from build123d import *

# Parameters (mm, degrees)
SKETCH_398_R        = 1.75
EXTRUDE_1_DEPTH     = 4
CHAMFER_1_SIZE      = 1.5
SKETCH_632_W        = 24
SKETCH_632_H        = 16
SKETCH_632_R        = 1.6
CUT_EXTRUDE_1_DEPTH = 3
SKETCH_910_R        = 2.5
SKETCH_910_W        = 7
SKETCH_910_H        = 4
EXTRUDE_2_DEPTH     = 1.2
SKETCH_1130_R       = 1.2
CUT_EXTRUDE_2_DEPTH = 0.7
CHAMFER_2_SIZE      = 1.2
CHAMFER_3_SIZE      = 2


with BuildPart() as part:
    # Sketch 398 → Бобышка-Вытянуть1 (new body)
    with BuildSketch(Plane(origin=(0, 0, 0), x_dir=(1, 0, 0), z_dir=(0, 1, 0))):
        with BuildLine():
            Line((-15, 4), (-13.5, 4))
            Line((-13.5, 4), (-13.5, 9.5))
            Line((-13.5, 9.5), (13.5, 9.5))
            Line((13.5, 9.5), (13.5, 4))
            Line((13.5, 4), (15, 4))
            ThreePointArc((15, 4), (19, 0), (15, -4))
            Line((15, -4), (13.5, -4))
            Line((13.5, -4), (13.5, -9.5))
            Line((13.5, -9.5), (-13.5, -9.5))
            Line((-13.5, -9.5), (-13.5, -4))
            Line((-13.5, -4), (-15, -4))
            ThreePointArc((-15, -4), (-19, 0), (-15, 4))
        make_face()
        with Locations((-15, 0)):
            Circle(SKETCH_398_R, mode=Mode.SUBTRACT)
        with Locations((15, 0)):
            Circle(SKETCH_398_R, mode=Mode.SUBTRACT)
    extrude(amount=EXTRUDE_1_DEPTH)

    # Фаска1
    chamfer_1_edges = [part.edges().sort_by_distance(p)[0] for p in [
        (13.25, 0, 0),
        (-16.75, 0, 0),
    ]]
    chamfer(chamfer_1_edges, length=CHAMFER_1_SIZE)

    # Sketch 632 → Вырез-Вытянуть1 (cut)
    with BuildSketch(Plane(origin=(0, 4, 0), x_dir=(1, 0, 0), z_dir=(0, 1, 0))):
        Rectangle(SKETCH_632_W, SKETCH_632_H)
        with Locations((-2.8, 4.2)):
            Circle(SKETCH_632_R, mode=Mode.SUBTRACT)
        with Locations((-2.8, -4.2)):
            Circle(SKETCH_632_R, mode=Mode.SUBTRACT)
    extrude(amount=-CUT_EXTRUDE_1_DEPTH, mode=Mode.SUBTRACT)

    # Sketch 910 → Бобышка-Вытянуть2 (add)
    with BuildSketch(Plane(origin=(0, 1, 0), x_dir=(1, 0, 0), z_dir=(0, 1, 0))):
        with Locations((-2.8, -4.2)):
            Circle(SKETCH_910_R)
        with Locations((-2.8, 4.2)):
            Circle(SKETCH_910_R)
        with Locations((8.5, -6)):
            Rectangle(SKETCH_910_W, SKETCH_910_H)
        with Locations((8.5, 6)):
            Rectangle(SKETCH_910_W, SKETCH_910_H)
    extrude(amount=EXTRUDE_2_DEPTH)

    # Sketch 1130 → Вырез-Вытянуть2 (cut)
    with BuildSketch(Plane(origin=(0, 1, 0), x_dir=(1, 0, 0), z_dir=(0, 1, 0))):
        with Locations((-8.3, 5.4)):
            Circle(SKETCH_1130_R)
    extrude(amount=-CUT_EXTRUDE_2_DEPTH, mode=Mode.SUBTRACT)

    # Фаска2
    chamfer_2_edges = [part.edges().sort_by_distance(p)[0] for p in [
        (12, 1, 0),
        (-3.5, 1, -8),
        (-12, 1, 0),
        (-3.5, 1, 8),
    ]]
    chamfer(chamfer_2_edges, length=CHAMFER_2_SIZE)

    # Фаска3
    chamfer_3_edges = [part.edges().sort_by_distance(p)[0] for p in [
        (0, 0, -9.5),
        (13.5, 0, -6.75),
        (13.5, 0, 6.75),
        (0, 0, 9.5),
        (-13.5, 0, 6.75),
        (-13.5, 0, -6.75),
    ]]
    chamfer(chamfer_3_edges, length=CHAMFER_3_SIZE)


solid = part.part
Read the model definition and answer for the solid it produces. Units are mm, in the model's axes. A direction names the side the tool comes from. Coordinates: 2 decimals unless noted, no trailing zeros. Order: outer loops, then holes, each group sorted by start corner. A loop starts at its lowest first (then second) coordinate and runs counter-clockwise, first axis right, second up. Notation, with made-up numbers: M 49.5,81.25 L 104.5,81.25 A19 cw 104.5,109.25 Z; hole C -6.75,-35 d7. An arc over 180 degrees is marked long. Put each result on its own line as item: value. Start each with the question number.
Item 1: Section A-A, the plane y = 2.55 is taken. Determine the outline of the cut face in (x, z), plus the area to 3 significant figures.
Item 2: Section D-D, the plane z = 0.5 is taken. Count the separate pieces of the cut face and the enclosed holes in it, plus the area to 3 significant figures.
Item 3: The mould has two halves that part along X. Classify faces 1 (the face through (5, 2, -6)), 2 (the face through (13.5, 3, -7)), 3 (the face through (-12.5, 1, -6.1)): +X half, -X half, draft (parallel to the pull), parting line (faces both ways), or undercut.
Item 4: Consider probe 1 along X at (y, z) = (2.25, 0); probe 2 along X at (y, z) = (2.25, 7); probe 3 along X at (y, z) = (1.55, -0.25). Determine where each line is inside the solid, lowest interval first. Write a range as [from, to].
Item 5: Section B-B, the plane x = -8.3 is taken. Determine the outline of the cut face in (y, z), plus the area to 3 significant figures.
Item 6: Section C-C, the plane z = -5.4 is taken. Determine the outline of the cut face in (x, y), plus the area to 3 significant figures.
Item 7: Given pin 1 Ø2 at (y, z) = (3, -7.5) entering from +X; pin 2 Ø1.4 at (y, z) = (3, 1) entering from -X; pin 3 Ø1.5 at (x, z) = (-3.5, -0.5) entering from +Y, each flat-ended and moving along its own axis, determine where each tip first touches the part or whether it passes through.
Item 8: For faces 4 (the face through (8, 2.2, 6)), 5 (the face through (-13.5, 3, -7)), 6 (the face through (0, 3, -9.5)), 7 (the face through (0, 3, 9.5)), 8 (the face through (-14, 2, 4)), determine the directions among +Z, -Z, +X, -X, +Y, -Y from which every point of the face is accessible in a straight line to the end or side of a thin tool.
Computed:
1. outline: M -15,-4 L -13.5,-4 L -13.5,-9.5 L 13.5,-9.5 L 13.5,-4 L 15,-4 A4 ccw 15,4 L 13.5,4 L 13.5,9.5 L -13.5,9.5 L -13.5,4 L -15,4 A4 ccw Z; C -2.8,-4.2 d3.2; C -2.8,4.2 d3.2; hole C -15,0 d3.5; hole M -12,-8 L 12,-8 L 12,8 L -12,8 Z; hole C 15,0 d3.5
1. area: 200 mm2
2. separate pieces: 3
2. enclosed holes: 0
2. area: 49.7 mm2
3. face 1: undercut
3. face 2: +X half
3. face 3: -X half
4. probe 1: x = [-19, -16.75], [-13.25, -12], [12, 13.25], [16.75, 19]
4. probe 2: x = [-13.5, -12], [12, 13.5]
4. probe 3: x = [-18.99, -16.73], [-13.27, -11.35], [11.35, 13.27], [16.73, 18.99]
5. outline: M 0,-7.5 L 2,-9.5 L 4,-9.5 L 4,-8 L 2.2,-8 L 1,-6.8 L 1,-6.6 L 0.3,-6.6 L 0.3,-4.2 L 1,-4.2 L 1,6.8 L 2.2,8 L 4,8 L 4,9.5 L 2,9.5 L 0,7.5 Z
5. area: 23.8 mm2
6. outline: M -13.5,2 L -11.5,0 L 11.5,0 L 13.5,2 L 13.5,4 L 12,4 L 12,2.2 L 5,2.2 L 5,1 L -0.61,1 L -0.61,2.2 L -1.74,2.2 L -1.74,4 L -3.86,4 L -3.86,2.2 L -4.99,2.2 L -4.99,1 L -7.1,1 L -7.1,0.3 L -9.5,0.3 L -9.5,1 L -10.8,1 L -12,2.2 L -12,4 L -13.5,4 Z
6. area: 48.5 mm2
7. pin 1: stops at x = 13.5
7. pin 2: stops at x = -18.99
7. pin 3: stops at y = 1
8. face 4: +Y
8. face 5: -Z, -X, +Y, -Y
8. face 6: -Z, +X, -X, +Y, -Y
8. face 7: +Z, +X, -X, +Y, -Y
8. face 8: +Z, -X, -Y
